Build history of the part. All positions in model axes, mm. Round coordinates to 2 decimals unless told otherwise and drop trailing zeros. Write each loop counter-clockwise with the first axis right and the second up, starting at its lowest first coordinate (ties: lowest second). Pieces come first, ordered by that corner, then holes.
1) Saw through at A-A (z = 27). Write the cut outline in (x, y).
2) Wall check: probe 1 along Y at (x, z) = (23.5, 67); probe 2 along Y at (x, z) = (-30, 49); probe 3 along X at (y, z) = (62, 63). Give the ranges that are in metal, low to high.
3) Flat gauge pins, fed straight in: pin 1 (2 mm diameter, centred on x = -81, z = 56.5, fed in from -Y); pin 2 (2 mm diameter, centred on x = 40.5, z = 60, fed in from +Y); pin 3 (10 mm diameter, centred on x = -36, z = 70.5, fed in from +Y). Where does each tip first touch, or does it go through?
4) Saw through at B-B (x = -68). Write the cut outline in (y, z).
5) Saw through at C-C (y = -74). Write the cut outline in (x, z), plus the area to 3 significant figures.
from build123d import *

# Parameters (mm, degrees)
F0_R     = 127
F1_DEPTH = 80
F2_R     = 105.6868422046
F3_DEPTH = 69.596
F4_R     = 105.629442308
F5_DEPTH = 67.31
F6_R     = 127
F6_R_2   = 105.6868422046
F7_DEPTH = 109.474
F8_R     = 105.6868422046
F9_DEPTH = 11.176


with BuildPart() as f1:
    # F0 (on Top) → F1 (new body)
    with BuildSketch(Plane.XY):
        Circle(F0_R)
    extrude(amount=F1_DEPTH)

    # F2 (on face) → F3 (cut)
    with BuildSketch(Plane.XY.offset(80)):
        Circle(F2_R)
    extrude(amount=-F3_DEPTH, mode=Mode.SUBTRACT)

    # F4 (on face) → F5 (join)
    with BuildSketch(Plane.XY.offset(10.404)):
        Circle(F4_R)
    extrude(amount=F5_DEPTH)

    # F6 (on face) → F7 (cut)
    with BuildSketch(Plane.XY.offset(80)):
        Circle(F6_R)
        Circle(F6_R_2, mode=Mode.SUBTRACT)
    extrude(amount=-F7_DEPTH, mode=Mode.SUBTRACT)

    # F8 (on face) → F9 (cut)
    with BuildSketch(Plane(origin=(0, 0, 0), x_dir=(1, 0, 0), z_dir=(0, 0, -1))):
        Circle(F8_R)
    extrude(amount=-F9_DEPTH, mode=Mode.SUBTRACT)


solid = f1.part
Evaluation:
1. outline: circle Ø211.26 at (0, 0)
2. probe 1: y = -102.98 to 102.98
2. probe 2: y = -101.28 to 101.28
2. probe 3: x = -85.52 to 85.52
3. pin 1: stops at y = -68.98
3. pin 2: stops at y = 97.97
3. pin 3: stops at y = 100.98
4. outline: (-80.83, 11.18) - (80.83, 11.18) - (80.83, 77.71) - (-80.83, 77.71) - close
5. outline: (-75.38, 11.18) - (75.38, 11.18) - (75.38, 77.71) - (-75.38, 77.71) - close
5. area: 10,000 mm2
